Can you work these out from the model? Positions are in its coordinate system, mm. A direction names the side the tool comes from. Give positions to 0.01 mm unless a question says otherwise; leave off trailing zeros. Write each loop counter-clockwise with the first axis right and the second up, starting at its lowest first coordinate (ties: lowest second). Pieces come first, ordered by that corner, then holes.
from build123d import *

# Parameters (mm, degrees)
F1_DEPTH = 38.1
F2_W     = 12.7
F2_H     = 6.35
F3_DEPTH = 25.401001


with BuildPart() as f1:
    # F0 (on Right) → F1 (new body)
    with BuildSketch(Plane.YZ):
        Polygon((0, 12.7), (0, 0), (25.400001, 0), (25.400001, 31.75), (12.700001, 31.75), (12.700001, 12.7), align=None)
    extrude(amount=F1_DEPTH)

    # F2 (on Front) → F3 (cut, through all)
    with BuildSketch(Plane.XZ):
        with Locations((18.293744, 28.697193)):
            Rectangle(F2_W, F2_H)
    extrude(amount=-F3_DEPTH, mode=Mode.SUBTRACT)


solid = f1.part
(1) Imagine slicing it at D-D, the plane z = 20.5. Write out the boundary of the cut face in (x, y).
Returned:
outline: (0, 12.7) - (38.1, 12.7) - (38.1, 25.4) - (0, 25.4) - close
(2) If I drill on L1, parallel to X at y = 17, z = 28; L2, parallel to Y at x = 16, z = 23; L3, parallel to Z at x = 17, y = 15.5, over which ranges is the centre line in solid material (lowest first)?
Returned:
L1: x = 0 to 11.94, 24.64 to 38.1
L2: y = 12.7 to 25.4
L3: z = 0 to 25.52
(3) Imagine slicing it at B-B, the plane y = 17. Write out the boundary of the cut face in (x, z).
Returned:
outline: (0, 0) - (38.1, 0) - (38.1, 31.75) - (24.64, 31.75) - (24.64, 25.52) - (11.94, 25.52) - (11.94, 31.75) - (0, 31.75) - close
(4) For faces 1 (the face through (18, 19, 25.522)), 2 (the face through (19, 25.4, 16)), 3 (the face through (19, 6, 12.7)), which set-ups out of +Z, -Z, +X, -X, +Y, -Y let a thin tool reach every point of the face, with its end or its side?
Returned:
face 1: +Z, +Y, -Y
face 2: +Z, -Z, +X, -X, +Y
face 3: +Z, +X, -X, -Y
(5) Imagine slicing it at A-A, the plane z = 27. Write out the boundary of the cut face in (x, y), plus the area to 3 significant figures.
Returned:
outline: (0, 12.7) - (11.94, 12.7) - (11.94, 25.4) - (0, 25.4) - close; (24.64, 12.7) - (38.1, 12.7) - (38.1, 25.4) - (24.64, 25.4) - close
area: 323 mm2
(6) If we mould it in two halves opening along X, with no side actions, what happens to faces 4 (the face through (11.944, 19, 29)), 5 (the face through (0, 15, 13)), 6 (the face through (38.1, 15, 13)), 7 (the face through (19, 13, 0))? For each: +X half, -X half, draft (parallel to the pull), parting line (faces both ways), or undercut.
Returned:
face 4: undercut
face 5: -X half
face 6: +X half
face 7: draft
(7) Imagine slicing it at C-C, the plane x = 18.5. Write out the boundary of the cut face in (y, z), plus the area to 3 significant figures.
Returned:
outline: (0, 0) - (25.4, 0) - (25.4, 25.52) - (12.7, 25.52) - (12.7, 12.7) - (0, 12.7) - close
area: 485 mm2
(8) Will these pins go through, and if not, where does the flat tip stop? P1, Ø5.5, axis at x = 10, z = 19.5, coming from the -Y side; P2, Ø4, axis at x = 24.5, y = 7, coming from the +Z side; P3, Ø8, axis at y = 6, z = 14.5, coming from the -X side.
Returned:
P1: stops at y = 12.7
P2: stops at z = 12.7
P3: stops at x = 0
